The listing builds one solid part. Answer for the finished solid, in the listing's coordinates (mm). A direction names the side the tool comes from. Give positions to 0.01 mm unless a question says otherwise; leave off trailing zeros. Loops run counter-clockwise (first coordinate to the right, second up) from the corner with the lowest first, then second, coordinate; pieces in that order, holes last. Notation, with made-up numbers: (84, 82.25) - (88, 82.25) arc R27 ccw to (88, 104.25) - close; hole circle Ø2 at (37, 68.25). An arc over 180 degrees is marked (long way). Write item = value, one per line. Start each with the question number.
1) The part is cut by section C-C on y = -57. Write down the section's boundary in (x, z), plus the area to 3 significant figures.
2) Consider probe 1 along Y at (x, z) = (36, 1.1); probe 2 along Y at (x, z) = (36, 1.45); probe 3 along Z at (x, y) = (41, -59.5). Determine where each line is inside the solid, lowest interval first.
3) The part is cut by section D-D on z = -7. Write down the section's boundary in (x, y).
4) Which of the six approach directions +Z, -Z, +X, -X, +Y, -Y give full straight-line access (tool end or side, diameter ignored) to faces 1 (the cylindrical face through (26.351, -118.711, -23.526)), 2 (the flat face through (-30.37, -48.36, 1.01)), 3 (the flat face through (-25.75, -106.2, -6.8))?
5) Flat-ended cylindrical pins translate along their axes: P1, Ø1.6, axis at y = -27, z = 0.5, coming from the +X side; P2, Ø1.6, axis at x = 2.5, z = 1, coming from the -Y side; P3, Ø0.6, axis at y = -18.5, z = 0.5, coming from the -X side. Find the tip coordinate at first contact, or state that the pin passes through.
6) The mould has two halves that part along X. Classify faces 4 (the flat face through (-29.37, -30.46, 1.01)), 5 (the flat face through (-63, -73.7, 0.5)), 6 (the flat face through (-44.11, -109.79, -12.55)): +X half, -X half, draft (parallel to the pull), parting line (faces both ways), or undercut.
7) The part is cut by section B-B on x = 53. Write down the section's boundary in (y, z).
8) The part is cut by section A-A on z = -17.5. Write down the section's boundary in (x, y).
from build123d import *
from OCP.BRepFilletAPI import BRepFilletAPI_MakeChamfer

# Parameters (mm, degrees)
BASE_FLANGE1_DEPTH      = 63
CUT_EXTRUDE1_DEPTH      = 138.978891404
CUT_EXTRUDE1_DEPTH_BACK = 138.978891404
SKETCH2_W               = 51.5
SKETCH2_H               = 35.5
FILLET1_R               = 2
CHAMFER1_SIZE           = 20
CHAMFER1_SIZE2          = 11.547005384
SKETCH3_R               = 1.3
CUT_EXTRUDE2_DEPTH      = 2
SKETCH4_W               = 2
SKETCH4_H               = 27
CUT_EXTRUDE3_DEPTH      = 2
FILLET2_R               = 2
CUT_EXTRUDE4_DEPTH      = 10
FILLET3_R               = 1


# Sheet-metal steps are written as plain solids
with BuildPart() as part:
    # Sketch1 → Base-Flange1 (new, symmetric)
    with BuildSketch(Plane(origin=(0, 0, 0), x_dir=(0, 0, -1), z_dir=(1, 0, 0))):
        with BuildLine():
            Line((0, 0), (0, -99.958865899))
            ThreePointArc((0, -99.958865899), (0.225978334, -100.882363125), (0.852847127, -101.597169987))
            Line((0.852847127, -101.597169987), (24.574561329, -118.207293091))
            Line((24.574561329, -118.207293091), (23.427408456, -119.845597179))
            Line((23.427408456, -119.845597179), (-0.294305745, -103.235474076))
            ThreePointArc((-0.294305745, -103.235474076), (-1.548043333, -101.805860352), (-2, -99.958865899))
            Line((-2, -99.958865899), (-2, 0))
            Line((-2, 0), (0, 0))
        make_face()
    extrude(amount=BASE_FLANGE1_DEPTH, both=True)

    # Sketch2 → Cut-Extrude1 (cut, two sides: drawn at the far end of the back side and taken through both)
    with BuildSketch(Plane.XY.offset(2).offset(-CUT_EXTRUDE1_DEPTH_BACK)):
        with Locations((0, -102.095597179)):
            Rectangle(SKETCH2_W, SKETCH2_H)
    extrude(amount=CUT_EXTRUDE1_DEPTH + CUT_EXTRUDE1_DEPTH_BACK, mode=Mode.SUBTRACT)

    # Fillet1
    fillet1_edges = [part.edges().sort_by_distance(p)[0] for p in [
        (-25.75, -84.345597179, 1),
        (25.75, -84.345597179, 1),
    ]]
    fillet(fillet1_edges, radius=FILLET1_R)

    # Chamfer1: one chamfer whose edges measure the first distance from different faces: ONE call of the kernel's chamfer builder (chamfer() names one face for all edges)
    chamfer1_edges_1 = [part.edges().sort_by_distance(p)[0] for p in [
        (63, -119.026445135, -24.000984892),
    ]]
    chamfer1_side_1 = [part.faces().sort_by_distance(p)[0] for p in [
        (44.375, -119.026445135, -24.000984892),
    ]]
    chamfer1_edges_2 = [part.edges().sort_by_distance(p)[0] for p in [
        (-63, -119.026445135, -24.000984892),
    ]]
    chamfer1_side_2 = [part.faces().sort_by_distance(p)[0] for p in [
        (-44.375, -119.026445135, -24.000984892),
    ]]
    chamfer1 = BRepFilletAPI_MakeChamfer(part.part.solid().wrapped)
    for e in chamfer1_edges_1:
        chamfer1.Add(CHAMFER1_SIZE, CHAMFER1_SIZE2, e.wrapped, chamfer1_side_1[0].wrapped)  # the first distance lies on this face
    for e in chamfer1_edges_2:
        chamfer1.Add(CHAMFER1_SIZE, CHAMFER1_SIZE2, e.wrapped, chamfer1_side_2[0].wrapped)  # the first distance lies on this face
    add(Compound.cast(chamfer1.Shape()), mode=Mode.REPLACE)

    # Sketch3 → Cut-Extrude2 (cut)
    with BuildSketch(Plane.XY.offset(2)):
        with Locations((-36, -14)):
            Circle(SKETCH3_R)
        with Locations((36, -14)):
            Circle(SKETCH3_R)
    extrude(amount=-CUT_EXTRUDE2_DEPTH, mode=Mode.SUBTRACT)

    # Sketch4 → Cut-Extrude3 (cut)
    with BuildSketch(Plane.XY.offset(2)):
        with Locations((-62, -13.5)):
            Rectangle(SKETCH4_W, SKETCH4_H)
        with Locations((62, -13.5)):
            Rectangle(SKETCH4_W, SKETCH4_H)
    extrude(amount=-CUT_EXTRUDE3_DEPTH, mode=Mode.SUBTRACT)

    # Fillet2
    fillet2_edges = [part.edges().sort_by_distance(p)[0] for p in [
        (63, -112.403354936, -14.542231827),
        (43, -119.026445135, -24.000984892),
        (25.75, -119.026445135, -24.000984892),
        (-63, -112.403354936, -14.542231827),
        (-43, -119.026445135, -24.000984892),
        (-25.75, -119.026445135, -24.000984892),
        (-63, -27, 1),
        (63, -27, 1),
        (61, 0, 1),
        (-61, 0, 1),
    ]]
    fillet(fillet2_edges, radius=FILLET2_R - 0.0001)  # a hair under: the kernel refuses the full size

    # Sketch5 → Cut-Extrude4 (cut)
    with BuildSketch(Plane.XY.offset(2)):
        Polygon((-40, -24.323383181), (-40, -30.096885873), (-20, -41.643891257), (-20, -35.870388565), align=None)
        Polygon((-40, -37.025089103), (-20, -48.572094487), (-20, -54.345597179), (-40, -42.798591795), align=None)
        Polygon((40, -42.798591795), (40, -37.025089103), (20, -48.572094487), (20, -54.345597179), align=None)
        Polygon((20, -35.870388565), (40, -24.323383181), (40, -30.096885873), (20, -41.643891257), align=None)
    extrude(amount=-CUT_EXTRUDE4_DEPTH, mode=Mode.SUBTRACT)

    # Fillet3
    fillet3_edges = [part.edges().sort_by_distance(p)[0] for p in [
        (-40, -42.798591795, 1),
        (-40, -37.025089103, 1),
        (-20, -48.572094487, 1),
        (-20, -54.345597179, 1),
        (40, -42.798591795, 1),
        (20, -54.345597179, 1),
        (20, -48.572094487, 1),
        (40, -37.025089103, 1),
        (20, -41.643891257, 1),
        (20, -35.870388565, 1),
        (40, -24.323383181, 1),
        (40, -30.096885873, 1),
        (-40, -24.323383181, 1),
        (-20, -35.870388565, 1),
        (-20, -41.643891257, 1),
        (-40, -30.096885873, 1),
    ]]
    fillet(fillet3_edges, radius=FILLET3_R)


solid = part.part
Answer below:
q1.outline = (-63, 0) - (63, 0) - (63, 2) - (-63, 2) - close
q1.area = 252 mm2
q2.probe_1 = -102.49 to -45.11, -39.33 to -32.41, -26.63 to -15.3, -12.7 to 0
q2.probe_2 = -101.98 to -45.11, -39.33 to -32.41, -26.63 to -15.3, -12.7 to 0
q2.probe_3 = 0 to 2
q3.outline = (-63, -108.34) - (-25.75, -108.34) - (-25.75, -105.9) - (-63, -105.9) - close; (25.75, -108.34) - (63, -108.34) - (63, -105.9) - (25.75, -105.9) - close
q4.face_1 = -Z, -Y
q4.face_2 = +Z, -Z
q4.face_3 = +Z, -Z, -Y
q5.P1 = 62.6
q5.P2 = -84.35
q5.P3 = -61
q6.face_4 = undercut
q6.face_5 = -X half
q6.face_6 = draft
q7.outline = (-116.53, -18.7) - (-114.9, -19.85) - (-101.6, -0.85) arc R2 cw to (-99.96, 0) - (0, 0) - (0, 2) - (-99.96, 2) arc R4 ccw to (-103.24, 0.29) - close
q8.outline = (-57.96, -113.25) - (-55.53, -115.7) - (-25.75, -115.7) - (-25.75, -113.25) - close; (25.75, -115.7) - (55.53, -115.7) - (57.96, -113.25) - (25.75, -113.25) - close
